Autodesk Inventor part; units mm, degrees
ref_plane "YZ Plane" through (0, 0, 0) normal (1, 0, 0) x (0, 1, 0)
ref_plane "XZ Plane" through (0, 0, 0) normal (0, 1, 0) x (-1, 0, 0)
ref_plane "XY Plane" through (0, 0, 0) normal (0, 0, 1) x (1, 0, 0)
sketch "Sketch1" plane through (0, 0, 0) normal (0, 0, 1) x (1, 0, 0)
  line L0 (-17.78, 0) -> (17.78, 0)
  line L1 (0, -17.78) -> (0, 17.78)
  line L2 (-12.7, 12.7) -> (12.7, 12.7)
  line L3 (12.7, 12.7) -> (12.7, -12.7)
  line L4 (12.7, -12.7) -> (-12.7, -12.7)
  line L5 (-12.7, -12.7) -> (-12.7, 12.7)
  line L6 (9.525, 9.525) -> (-9.525, 9.525)
  line L7 (-9.525, 9.525) -> (-9.525, -9.525)
  line L8 (-9.525, -9.525) -> (9.525, -9.525)
  line L9 (9.525, -9.525) -> (9.525, 9.525)
  point P0 (0, 0)
  point P1 (-12.7, 0)
  point P2 (0, 12.7)
  dimension "d0" = 25.4
  dimension "d1" = 3.175
extrude "Extrusion1" add sketch "Sketch1" along normal mid plane 403.225 contours L5 L2 L1 L6 L7 L0 | L0 L7 L8 L1 L4 L5 | L1 L8 L9 L0 L3 L4 | L2 L3 L0 L9 L6 L1
sketch "Sketch3" plane through (-12.7, 12.7, 201.6125) normal (0, 1, 0) x (1, 0, 0)
  line L0 (0, 0) -> (25.4, 0)
  line L1 (25.4, 0) -> (25.4, 403.225)
  line L2 (0, 0) -> (25.4, 25.4)
  point P0 (12.7, 201.6125)
  dimension "d7" = 45
extrude "Extrusion3" cut sketch "Sketch3" against normal through all
sketch "Sketch4" plane through (-12.7, 12.7, -201.6125) normal (0, 1, 0) x (1, 0, 0)
  line L0 (25.4, -377.825) -> (25.4, 0)
  line L1 (25.4, 0) -> (0, 0)
  line L2 (0, 0) -> (25.4, -25.4)
  point P0 (12.7, -201.6125)
  dimension "d10" = 45
extrude "Extrusion4" cut sketch "Sketch4" against normal through all
properties part number "tubing_template_0.125" material "Aluminum-6061"
Source: CAD feature listing. Evaluate the final solid. Frame: model axes, mm. A direction names the side the tool comes from. Coordinates: 2 decimals unless noted, no trailing zeros. Loops run counter-clockwise (first coordinate to the right, second up) from the corner with the lowest first, then second, coordinate; pieces in that order, holes last. Notation, with made-up numbers: (-30, 24) -> (-8, 24) arc R20 cw to (-8, 59) -> close; hole circle Ø5 at (4.25, -32.5). An arc over 180 degrees is marked (long way). Answer in a Markdown table with one row per item. Add a question column.
Q1. Section B-B on x = 2.25. Return the cut outline in (y, z) (1 decimal), and give its area (3 significant figures).
Q2. Section C-C on z = -22. Return the cut outline in (x, y) (3 decimals).
Q3. Pull-direction query (Y, two-part tool) for faces 1 (the face through (-12.7, 0, -3)), 2 (the face through (0, -12.7, -3)), 3 (the face through (9.525, 0, -3)); classes: pulls with the +Y half, pulls with the -Y half, needs draft (parallel to the pull), parting line crosses it, or undercut.
Q4. Contact query for flat-ended pins moving along their axis: pin 1 Ø1.5 at (x, y) = (9, -5) entering from -Z; pin 2 Ø8 at (x, y) = (-9.5, -0.5) entering from -Z; pin 3 Ø6 at (x, y) = (-4.5, -9) entering from +Z. Output: stop coordinate, or through.
Q5. Section A-A on y = 0.25. Return the cut outline in (x, z) (1 decimal), and give its area (3 significant figures).
Q6. Ray query, line 1 along Y through (x, z) = (-4.25, -10) (3 decimals); line 2 along Z through (x, y) = (5.5, 11.75). Return the intervals inside material, ascending.
Q7. Reachability of faces 4 (the face through (-0.18, -11.11, 189.09)), 5 (the face through (0, -9.525, -3)) from +Z, -Z, +X, -X, +Y, -Y: full face, straight path, thin tool, end or side. Return the list, or none.
Computed values:
| question | item | result |
|---|---|---|
| 1 | outline | (-12.7, -186.7) -> (-9.5, -186.7) -> (-9.5, 186.7) -> (-12.7, 186.7) -> close; (9.5, -186.7) -> (12.7, -186.7) -> (12.7, 186.7) -> (9.5, 186.7) -> close |
| 1 | area | 2,370 mm^2 |
| 2 | outline | (-12.7, -12.7) -> (12.7, -12.7) -> (12.7, 12.7) -> (-12.7, 12.7) -> close; hole (-9.525, -9.525) -> (9.525, -9.525) -> (9.525, 9.525) -> (-9.525, 9.525) -> close |
| 3 | face 1 | needs draft |
| 3 | face 2 | pulls with the -Y half |
| 3 | face 3 | undercut |
| 4 | pin 1 | stops at z = -179.39 |
| 4 | pin 2 | stops at z = -201.61 |
| 4 | pin 3 | stops at z = 196.37 |
| 5 | outline | (-12.7, -201.6) -> (-9.5, -198.4) -> (-9.5, 198.4) -> (-12.7, 201.6) -> close; (9.5, -179.4) -> (12.7, -176.2) -> (12.7, 176.2) -> (9.5, 179.4) -> close |
| 5 | area | 2,400 mm^2 |
| 6 | line 1 | y = -12.7 to -9.525, 9.525 to 12.7 |
| 6 | line 2 | z = -183.41 to 183.41 |
| 7 | face 4 | +Z, +X, +Y, -Y |
| 7 | face 5 | +Z, -Z |
